Autodesk Inventor part; units mm, degrees
ref_plane "YZ Plane" through (0, 0, 0) normal (1, 0, 0) x (0, 1, 0)
ref_plane "XZ Plane" through (0, 0, 0) normal (0, 1, 0) x (-1, 0, 0)
ref_plane "XY Plane" through (0, 0, 0) normal (0, 0, 1) x (1, 0, 0)
sketch "スケッチ1" plane through (0, 0, 0) normal (0, 1, 0) x (-1, 0, 0)
  circle A0 centre (0, 0) radius 57.5
  circle A1 centre (0, 0) radius 70
  dimension "d0" = 115
  dimension "d1" = 140
extrude "押し出し1" add sketch "スケッチ1" along normal blind 8.5
sketch "スケッチ2" plane through (0, 8.5, 0) normal (0, 1, 0) x (1, 0, 0)
  point P0 (0, 0)
  point P1 (0, 64)
  point P2 (-64, 0)
  point P3 (0, -64)
  point P4 (64, 0)
  dimension "d4" = 64
  dimension "d7" = 360
hole "穴1" at (0, 8.5, -64) at (-64, 8.5, 0) at (0, 8.5, 64) at (64, 8.5, 0) direction (0, -1, 0) diameter 5 end through all
properties part number "turntable2" material "アルミニウム 6061"
Source: CAD feature listing. Evaluate the final solid. Frame: model axes, mm. Round coordinates to 2 decimals unless told otherwise and drop trailing zeros. Loops run counter-clockwise (first coordinate to the right, second up) from the corner with the lowest first, then second, coordinate; pieces in that order, holes last.
Q1. Section D-D, the plane y = 2.5. Return loops of the section in (x, z), plus the area to 3 significant figures.
Q2. First-contact query: P1, Ø10, axis at x = -56, z = -48, coming from the -Y side; P2, Ø2, axis at x = 24, y = 4.5, coming from the -Z side; P3, Ø5, axis at x = 13.5, y = 5.5, coming from the +Z side; P4, Ø3, axis at y = 7.5, z = -33.5, coming from the +X side. Flat tips, straight axial feed; report the tip coordinate or a pass-through.
Q3. Mould query, pull axis Z, two halves, no side actions, for faces 1 (the face through (0.96, 4.19, -61.69)), 2 (the face through (-26, 8.5, -52)), 3 (the face through (55.55, 4.19, 42.594)). Classes: pulls with the +Z half, pulls with the -Z half, needs draft (parallel to the pull), parting line crosses it, or undercut.
Q4. Section A-A, the plane z = 0. Return loops of the section in (x, y).
Q5. Section C-C, the plane x = 19.5. Return loops of the section in (y, z).
Q6. Ray query, line 1 (Z direction, x = 0, y = 3.75); line 2 (X direction, y = 4.5, z = 1.5); line 3 (Z direction, x = -27.5, y = 5.5). Return the intervals inside material, ascending.
Q7. Section B-B, the plane x = 0. Return loops of the section in (y, z), plus the area to 4 significant figures.
Solutions:
1. outline: circle Ø140 at (0, 0); hole circle Ø5 at (-64, 0); hole circle Ø115 at (0, 0); hole circle Ø5 at (0, -64); hole circle Ø5 at (0, 64); hole circle Ø5 at (64, 0)
1. area: 4,930 mm2
2. P1: stops at y = 0
2. P2: stops at z = -66.11
2. P3: stops at z = 69.13
2. P4: stops at x = 62.26
3. face 1: undercut
3. face 2: needs draft
3. face 3: parting line crosses it
4. outline: (-70, 0) - (-66.5, 0) - (-66.5, 8.5) - (-70, 8.5) - close; (-61.5, 0) - (-57.5, 0) - (-57.5, 8.5) - (-61.5, 8.5) - close; (57.5, 0) - (61.5, 0) - (61.5, 8.5) - (57.5, 8.5) - close; (66.5, 0) - (70, 0) - (70, 8.5) - (66.5, 8.5) - close
5. outline: (0, -67.23) - (8.5, -67.23) - (8.5, -54.09) - (0, -54.09) - close; (0, 54.09) - (8.5, 54.09) - (8.5, 67.23) - (0, 67.23) - close
6. line 1: z = -70 to -66.5, -61.5 to -57.5, 57.5 to 61.5, 66.5 to 70
6. line 2: x = -69.98 to -66, -62 to -57.48, 57.48 to 62, 66 to 69.98
6. line 3: z = -64.37 to -50.5, 50.5 to 64.37
7. outline: (0, -70) - (8.5, -70) - (8.5, -66.5) - (0, -66.5) - close; (0, -61.5) - (8.5, -61.5) - (8.5, -57.5) - (0, -57.5) - close; (0, 57.5) - (8.5, 57.5) - (8.5, 61.5) - (0, 61.5) - close; (0, 66.5) - (8.5, 66.5) - (8.5, 70) - (0, 70) - close
7. area: 127.5 mm2
